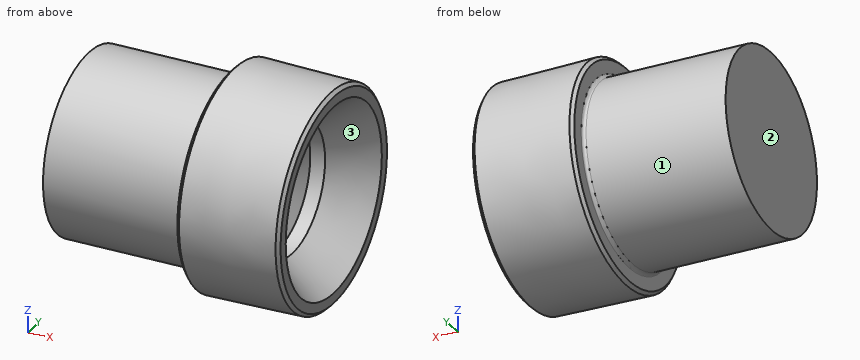
Autodesk Inventor part; units mm, degrees
ref_plane "YZ Plane" through (0, 0, 0) normal (1, 0, 0) x (0, 1, 0)
ref_plane "XZ Plane" through (0, 0, 0) normal (0, 1, 0) x (-1, 0, 0)
ref_plane "XY Plane" through (0, 0, 0) normal (0, 0, 1) x (1, 0, 0)
sketch "Sketch1" plane through (0, 0, 0) normal (0, 0, 1) x (1, 0, 0)
  line L0 (0, 0) -> (0, 6.9469)
  line L1 (0, 6.9469) -> (10.8458, 6.9469)
  line L2 (11.0998, 7.2009) -> (11.0998, 8.2277)
  line L3 (11.3538, 8.4772) -> (18.796, 8.3473)
  line L4 (19.05, 8.0889) -> (19.05, 7.3025)
  line L5 (19.05, 7.3025) -> (15.8337, 4.9657)
  line L6 (15.8337, 4.9657) -> (14.6812, 4.9657)
  line L7 (0, 0) -> (11.6975, 0)
  line L8 (11.6975, 0) -> (14.6812, 4.9657)
  arc A0 (10.8458, 6.9469) -> (11.0998, 7.2009) centre (10.8458, 7.2009) ccw
  line L9 (19.05, 8.0889) -> (18.796, 8.3473)
  line L10 (11.0998, 8.2277) -> (11.3538, 8.4772)
  point P0 (11.0998, 6.9469)
  point P1 (11.0998, 8.4817)
  point P2 (19.05, 8.3429)
  dimension "d0" = 6.9469
  dimension "d1" = 8.6741
  dimension "d2" = 7.9502
  dimension "d3" = 19.05
  dimension "d4" = 4.9657
  dimension "d5" = 4.3688
  dimension "d6" = 37
  dimension "d7" = 7.3025
  dimension "d8" = 59
  dimension "d11" = 0.254
  dimension "d12" = 0.254
  dimension "d13" = 0.254
  dimension "d14" = 0.254
  dimension "d15" = 0.254
  dimension "d16" = 1
revolve "Revolution1" add sketch "Sketch1" angle 360 about axis through (0, 0, 0) along (1, 0, 0)
equation "\"d0\" = 0.5 * AN929_C"
equation "\"d1\" = 0.5 * AN929_B"
equation "\"d2\" = AN929_D"
equation "\"d3\" = AN929_H"
equation "\"d4\" = 0.5 * AN929_F"
equation "\"d5\" = AN929_E"
equation "\"d7\" = 0.5 * AN929_G"
equation "\"d11\" = AN929_R"
equation "\"Tube_OD\" = 12.7"
equation "\"AN929_B\" = 17.3482"
equation "\"AN929_C\" = 13.8938"
equation "\"AN929_D\" = 7.9502"
equation "\"AN929_E\" = 4.3688"
equation "\"AN929_F\" = 9.9314"
equation "\"AN929_G\" = 14.605"
equation "\"AN929_H\" = 19.05"
equation "\"AN929_R\" = 0.254"
properties part number "AN929-8D" material "Aluminum 2014-T6"
Part model, mm, in its own coordinate system. Face numbers are marked on the shaded views. Round coordinates to 2 decimals unless told otherwise and drop trailing zeros. Order: outer loops, then holes, each group sorted by start corner. A loop starts at its lowest first (then second) coordinate and runs counter-clockwise, first axis right, second up. Notation, with made-up numbers: M 37,45.5 L 47,45.5 A29 cw 47,70.5 Z; hole C -23,45 d9. An arc over 180 degrees is marked long. Answer in a Markdown table with one row per item. Add a question column.
Q1. Mould opens along Z. For the marked faces 1, 2 and 3 say: +Z half, -Z half, draft (parallel to the pull), parting line (faces both ways), or undercut.
Q2. Cut at A-A on x = 1.5. Give the cut face in (y, z), and give its area (3 significant figures).
Q3. Pin check, flat tips, straight feed: pin 1 (1.5 mm diameter, centred on x = 15.5, y = -5, fed in from -Z); pin 2 (1.5 mm diameter, centred on x = 14, y = 1.5, fed in from -Z); pin 3 (2 mm diameter, centred on y = 5, z = -1, fed in from +X). Stop position of each tip, or through.
Q4. Wall check: L1, parallel to X at y = -2.25, z = 7.5; L2, parallel to Z at x = 15.3, y = 0; L3, parallel to Z at x = 2.25, y = 0.5. Give the ranges that are in metal, low to high. Write a range as from..to.
Established:
| question | item | result |
|---|---|---|
| 1 | face 1 | parting line |
| 1 | face 2 | draft |
| 1 | face 3 | undercut |
| 2 | outline | C 0,0 d13.89 |
| 2 | area | 152 mm2 |
| 3 | pin 1 | stops at z = -7.25 |
| 3 | pin 2 | stops at z = -8.4 |
| 3 | pin 3 | stops at x = 17.39 |
| 4 | L1 | x = 11.1..19.05 |
| 4 | L2 | z = -8.41..-4.97, 4.97..8.41 |
| 4 | L3 | z = -6.93..6.93 |
